Verification items for the finished model (mm, model axes). A direction names the side the tool comes from. Give positions to 0.01 mm unless a question says otherwise; leave off trailing zeros. Write each loop counter-clockwise with the first axis right and the second up, starting at its lowest first coordinate (ties: lowest second). Pieces come first, ordered by that corner, then holes. Notation, with made-up numbers: (48, -33) -> (66, -33) arc R32 cw to (66, -2) -> close; hole circle Ø9 at (0.5, 85.25). An arc over 180 degrees is marked (long way). Write item = value, one per line.
Autodesk Inventor part; units mm, degrees
ref_plane "YZ Plane" through (0, 0, 0) normal (1, 0, 0) x (0, 1, 0)
ref_plane "XZ Plane" through (0, 0, 0) normal (0, 1, 0) x (-1, 0, 0)
ref_plane "XY Plane" through (0, 0, 0) normal (0, 0, 1) x (1, 0, 0)
sketch "Sketch20" plane through (0, 0, 0) normal (1, 0, 0) x (0, 1, 0)
  line L0 (-1.0403, 3.8823) -> (-51.7638, 193.1852)
  line L1 (0, 0) -> (195.9808, 0) construction
  line L2 (-1.0403, -3.8823) -> (-51.7638, -193.1852)
  line L3 (0, 0) -> (200, 0) construction
  arc A0 (-1.0403, -3.8823) -> (-1.0403, 3.8823) centre (-15.5291, 0) ccw
  line L4 (-50.7979, 193.444) -> (-0.0743, 4.1411)
  arc A1 (-0.0743, -4.1411) -> (-0.0743, 4.1411) centre (-15.5291, 0) ccw
  line L5 (-0.0743, -4.1411) -> (-50.7979, -193.444)
  line L6 (-50.7979, 193.444) -> (-51.7638, 193.1852)
  line L7 (-50.7979, -193.444) -> (-51.7638, -193.1852)
  dimension "d97" = 90
  dimension "d81" = 200
  dimension "d82" = 105
  dimension "d83" = 200
  dimension "d84" = 105
  dimension "d85" = 15
  dimension "d86" = 1
  dimension "d87" = 90
  dimension "d88" = 90
extrude "Extrusion7" add sketch "Sketch20" along normal blind 400
sketch "Sketch21" plane through (0, 0, 0) normal (0, 0, 1) x (1, 0, 0)
  line L0 (0, -51.7638) -> (0, -1.0403)
  line L1 (0, -51.7638) -> (196.1177, 0.7858)
  line L2 (0, -51.7638) -> (210, -51.7638) construction
  line L3 (400, -50.7979) -> (400, -51.7638)
  line L4 (400, -51.7638) -> (203.8823, 0.7858)
  line L5 (400, -51.7638) -> (610, -51.7638) construction
  arc A0 (203.8823, 0.7858) -> (196.1177, 0.7858) centre (200, -13.7031) ccw
  line L6 (400, -51.7638) -> (400, 8.2362)
  line L7 (400, -0.0743) -> (400, -50.7979)
  line L8 (400, -51.7638) -> (460, -51.7638) construction
  line L9 (0, -51.7638) -> (0, 8.2362)
  line L10 (400, 8.2362) -> (0, 8.2362)
  point P0 (0, 0)
  dimension "d92" = 15
  dimension "d94" = 165
  dimension "d95" = 15
  dimension "d96" = 60
  dimension "d97" = 90
extrude "Extrusion8" cut sketch "Sketch21" along normal through all both and the other way through all
sketch "Sketch22" plane through (210.6971, -1.0403, 3.8823) normal (0.2588, 0.9659, 0) x (0.6947, -0.1862, 0.6947)
  line L0 (272.4776, 0) -> (269.9731, -2.779)
  line L1 (0, 0) -> (272.4776, 0)
  ellipse E0 centre (37.5672, 41.6848) end of major axis (79.252, 81.9492) minor radius 15 (-5.3944, 5.5847) -> (0, 0) ccw
  line L2 (4.0481, 277.8986) -> (-5.3944, 5.5847)
  line L3 (1.184, 275.492) -> (4.0481, 277.8986)
  line L4 (-8.2585, 3.178) -> (1.184, 275.492)
  ellipse E1 centre (37.5672, 41.6848) end of major axis (-6.8966, -1.2639) minor radius 16 (-8.2585, 3.178) -> (-2.5045, -2.779) ccw
  line L5 (269.9731, -2.779) -> (-2.5045, -2.779)
  line L6 (4.0481, 277.8986) -> (-5.3944, 5.5847)
  line L7 (4.0481, 277.8986) -> (272.4776, 0)
  point P0 (-149.272, -138.788)
extrude "Extrusion9" add sketch "Sketch22" along normal blind 1 contours L1 E0 L2 L7
sketch "Sketch24" plane through (0, -51.7638, 193.1852) normal (-0.2588, 0.9659, 0) x (0.6947, 0.1862, -0.6947)
  line L0 (0, 0) -> (272.4776, 0)
  line L1 (2.5045, -2.779) -> (0, 0)
  line L2 (274.9821, -2.779) -> (2.5045, -2.779)
  ellipse E0 centre (234.9104, 41.6848) end of major axis (279.3742, -1.2639) minor radius 16 (274.9821, -2.779) -> (280.7361, 3.178) ccw
  line L3 (271.2936, 275.492) -> (280.7361, 3.178)
  line L4 (268.4295, 277.8986) -> (271.2936, 275.492)
  line L5 (277.872, 5.5847) -> (268.4295, 277.8986)
  ellipse E1 centre (234.9104, 41.6848) end of major axis (193.2256, 81.9492) minor radius 15 (272.4776, 0) -> (277.872, 5.5847) ccw
  line L6 (277.872, 5.5847) -> (268.4295, 277.8986)
  line L7 (268.4295, 277.8986) -> (0, 0)
  point P0 (143.8509, 129.6415)
extrude "Extrusion10" add sketch "Sketch24" along normal blind 1 contours L7 L5 E1 L0
equation "\"BendRadius\" = Thickness"
equation "\"BendReliefWidth\" = Thickness"
equation "\"BendReliefDepth\" = 0.5 * Thickness"
equation "\"CornerReliefSize\" = 4 * Thickness"
equation "\"MinimumRemnant\" = 2 * Thickness"
equation "\"TransitionRadius\" = BendRadius"
equation "\"JacobiRadiusSize\" = Thickness"
equation "\"GapSize\" = Thickness"
properties part number "chimneyRoof"
Item 1: Sectioned sample at C-C on y = -36.5. Record the cut outline in (x, z).
Response values:
outline = (53.1, -139.83) -> (56.97, -136.22) -> (56.97, -140.08) -> (343.03, -140.08) -> (343.03, -136.22) -> (346.9, -139.83) -> (346.9, 139.82) -> (343.03, 136.22) -> (343.03, -136.22) -> (56.97, -136.22) -> (56.97, 136.22) -> (343.03, 136.22) -> (343.03, 140.08) -> (56.97, 140.08) -> (56.97, 136.22) -> (53.1, 139.83) -> close
Item 2: Set-up check for faces 5 (the flat face through (304.152, -25.571, 97.208)), 6 (the flat face through (64.25, -34.55, -24.02)), 7 (the flat face through (306.8, -26.28, -99.86)), 8 (the flat face through (63.991, -33.582, -24.021)): record each of +Z, -Z, +X, -X, +Y, -Y from which the full face is reachable in a straight line by a thin tool's end or side.
Response values:
face_5 = +Z, +Y
face_6 = -Y
face_7 = -Z, +Y
face_8 = +Z, -Z, -X, +Y
Item 3: Sectioned sample at D-D on z = -143.5. Record the cut outline in (x, y).
Response values:
outline = (-0.26, -50.8) -> (0, -51.76) -> (49.69, -38.45) -> (350.31, -38.45) -> (400, -51.76) -> (400.26, -50.8) -> (350.57, -37.48) -> (350.31, -38.45) -> (346.45, -37.42) -> (53.55, -37.42) -> (49.69, -38.45) -> (49.43, -37.48) -> close
Item 4: Go/stop test with flat-tipped pins: P1, Ø1.5, axis at x = 140.5, z = 30, coming from the +Y side; P2, Ø10, axis at x = 285, y = -14, coming from the +Z side; P3, Ø4, axis at x = 162.5, z = -95, coming from the -Y side; P4, Ø1, axis at x = 160.5, z = -20.5, coming from the +Y side. Record where each tip stops, or that it passes through.
Response values:
P1 = -12.88
P2 = through
P3 = -25.99
P4 = -7.59
Item 5: Material ranges on line 1 (Y direction, x = 193, z = 86); line 2 (Y direction, x = 132, z = -50), recorded low to high.
Response values:
line_1 = -23.04 to -22.01
line_2 = -16.39 to -15.36
Item 6: Mould release check, pull along Z, two halves, no side actions. Record for faces 1 (the flat face through (197.2, -31.683, -118.242)), 2 (the flat face through (354.759, -38.606, -5.276)), 3 (the flat face through (197.25, -31.427, 121.151)), 4 (the flat face through (354.499, -39.572, -5.275)): +Z half, -Z half, draft (parallel to the pull), parting line (faces both ways), or undercut.
Response values:
face_1 = undercut
face_2 = draft
face_3 = +Z half
face_4 = undercut
Item 7: Sectioned sample at B-B on x = 275. Record the cut outline in (y, z) (3 decimals).
Response values:
outline = (-51.764, -193.185) -> (-50.798, -193.444) -> (-18.27, -72.049) -> (-18.27, -68.187) -> (-17.235, -67.928) -> (-17.235, 67.925) -> (-18.27, 68.184) -> (-18.27, -68.185) -> close; (-51.764, 193.185) -> (-18.27, 68.185) -> (-18.27, 72.049) -> (-50.798, 193.444) -> close
Item 8: Sectioned sample at A-A on z = 73.5. Record the cut outline in (x, y), then the cut area to 3 significant figures.
Response values:
outline = (-0.26, -50.8) -> (0, -51.76) -> (119.69, -19.69) -> (280.31, -19.69) -> (276.45, -18.66) -> (123.55, -18.66) -> (119.69, -19.69) -> (119.43, -18.73) -> close; (280.32, -19.69) -> (400, -51.76) -> (400.26, -50.8) -> (280.58, -18.73) -> close
area = 410 mm^2
